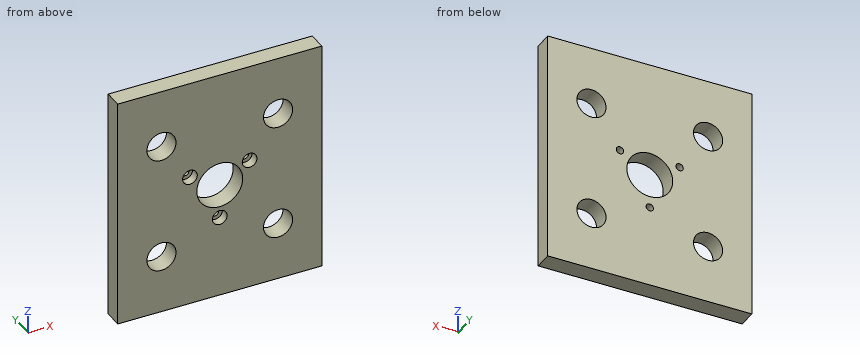
```python
from build123d import *

# Parameters (mm, degrees)
SKETCH1_W           = 44.45
SKETCH1_H           = 50.8
SKETCH1_R           = 0.8
SKETCH1_R_2         = 5
SKETCH1_R_3         = 3.175
BOSS_EXTRUDE1_DEPTH = 4
SKETCH2_R           = 1.6
CUT_EXTRUDE2_DEPTH  = 2


with BuildPart() as part:
    # Sketch1 → Boss-Extrude1 (new body)
    with BuildSketch(Plane(origin=(0, 0, 0), x_dir=(1, 0, 0), z_dir=(0, 1, 0))):
        Rectangle(SKETCH1_W, SKETCH1_H)
        with Locations(Location((0, 7.5, 0), (0, 0, 270))):
            Circle(SKETCH1_R, mode=Mode.SUBTRACT)
        with Locations(Location((6.495190528, -3.75, 0), (0, 0, 270))):
            Circle(SKETCH1_R, mode=Mode.SUBTRACT)
        with Locations(Location((-6.495190528, -3.75, 0), (0, 0, 270))):
            Circle(SKETCH1_R, mode=Mode.SUBTRACT)
        with Locations(Location((0, 0, 0), (0, 0, 270))):
            Circle(SKETCH1_R_2, mode=Mode.SUBTRACT)
        with Locations(Location((-12.7, 12.7, 0), (0, 0, 270))):
            Circle(SKETCH1_R_3, mode=Mode.SUBTRACT)
        with Locations(Location((-12.7, -12.7, 0), (0, 0, 270))):
            Circle(SKETCH1_R_3, mode=Mode.SUBTRACT)
        with Locations(Location((12.7, -12.7, 0), (0, 0, 270))):
            Circle(SKETCH1_R_3, mode=Mode.SUBTRACT)
        with Locations(Location((12.7, 12.7, 0), (0, 0, 270))):
            Circle(SKETCH1_R_3, mode=Mode.SUBTRACT)
    extrude(amount=BOSS_EXTRUDE1_DEPTH)

    # Sketch2 → Cut-Extrude2 (cut)
    with BuildSketch(Plane(origin=(0, 0, 0), x_dir=(1, 0, 0), z_dir=(0, 1, 0))):
        with Locations(Location((6.495190528, -3.75, 0), (0, 0, 270))):
            Circle(SKETCH2_R)
        with Locations(Location((-6.495190528, -3.75, 0), (0, 0, 270))):
            Circle(SKETCH2_R)
        with Locations(Location((0, 7.5, 0), (0, 0, 270))):
            Circle(SKETCH2_R)
    extrude(amount=CUT_EXTRUDE2_DEPTH, mode=Mode.SUBTRACT)


solid = part.part
```
Here's how the part is built. I have some questions about the finished solid (model axes, mm). Coordinates: 2 decimals unless noted, no trailing zeros. Order: outer loops, then holes, each group sorted by start corner. A loop starts at its lowest first (then second) coordinate and runs counter-clockwise, first axis right, second up.
1) Will these pins go through, and if not, where does the flat tip stop? pin 1 (2 mm diameter, centred on x = -6.5, z = 3.75, fed in from -Y); pin 2 (5.5 mm diameter, centred on x = -12.7, z = 12.7, fed in from +Y).
2) Imagine slicing it at B-B on z = -12.7. List the corners of the cut face in (x, y) for me (3 decimals), and give its area (3 significant figures).
3) I need wall thicknesses on line 1 (X direction, y = 3.1, z = -12.7) (3 decimals); line 2 (X direction, y = 2.05, z = 0) (3 decimals); line 3 (X direction, y = 2.2, z = 14) (3 decimals). Which ranges of each line are inside material? Lowest first, please.
4) Imagine slicing it at A-A on x = 0. List the corners of the cut face in (y, z) for me, and give its area (3 significant figures).
5) Imagine slicing it at D-D on x = -12.7. List the corners of the cut face in (y, z) for me (3 decimals), and give its area (3 significant figures).
6) Imagine slicing it at C-C on z = 0. List the corners of the cut face in (x, y) for me (3 decimals), and give its area (3 significant figures).
Response values:
1. pin 1: stops at y = 2
1. pin 2: passes through
2. outline: (-22.225, 0) - (-15.875, 0) - (-15.875, 4) - (-22.225, 4) - close; (-9.525, 0) - (9.525, 0) - (9.525, 4) - (-9.525, 4) - close; (15.875, 0) - (22.225, 0) - (22.225, 4) - (15.875, 4) - close
2. area: 127 mm2
3. line 1: x = -22.225 to -15.875, -9.525 to 9.525, 15.875 to 22.225
3. line 2: x = -22.225 to -5, 5 to 22.225
3. line 3: x = -22.225 to -15.597, -9.803 to 9.803, 15.597 to 22.225
4. outline: (0, -25.4) - (4, -25.4) - (4, -8.3) - (2, -8.3) - (2, -9.1) - (0, -9.1) - close; (0, -5.9) - (2, -5.9) - (2, -6.7) - (4, -6.7) - (4, -5) - (0, -5) - close; (0, 5) - (4, 5) - (4, 25.4) - (0, 25.4) - close
4. area: 154 mm2
5. outline: (0, -25.4) - (4, -25.4) - (4, -15.875) - (0, -15.875) - close; (0, -9.525) - (4, -9.525) - (4, 9.525) - (0, 9.525) - close; (0, 15.875) - (4, 15.875) - (4, 25.4) - (0, 25.4) - close
5. area: 152 mm2
6. outline: (-22.225, 0) - (-5, 0) - (-5, 4) - (-22.225, 4) - close; (5, 0) - (22.225, 0) - (22.225, 4) - (5, 4) - close
6. area: 138 mm2
